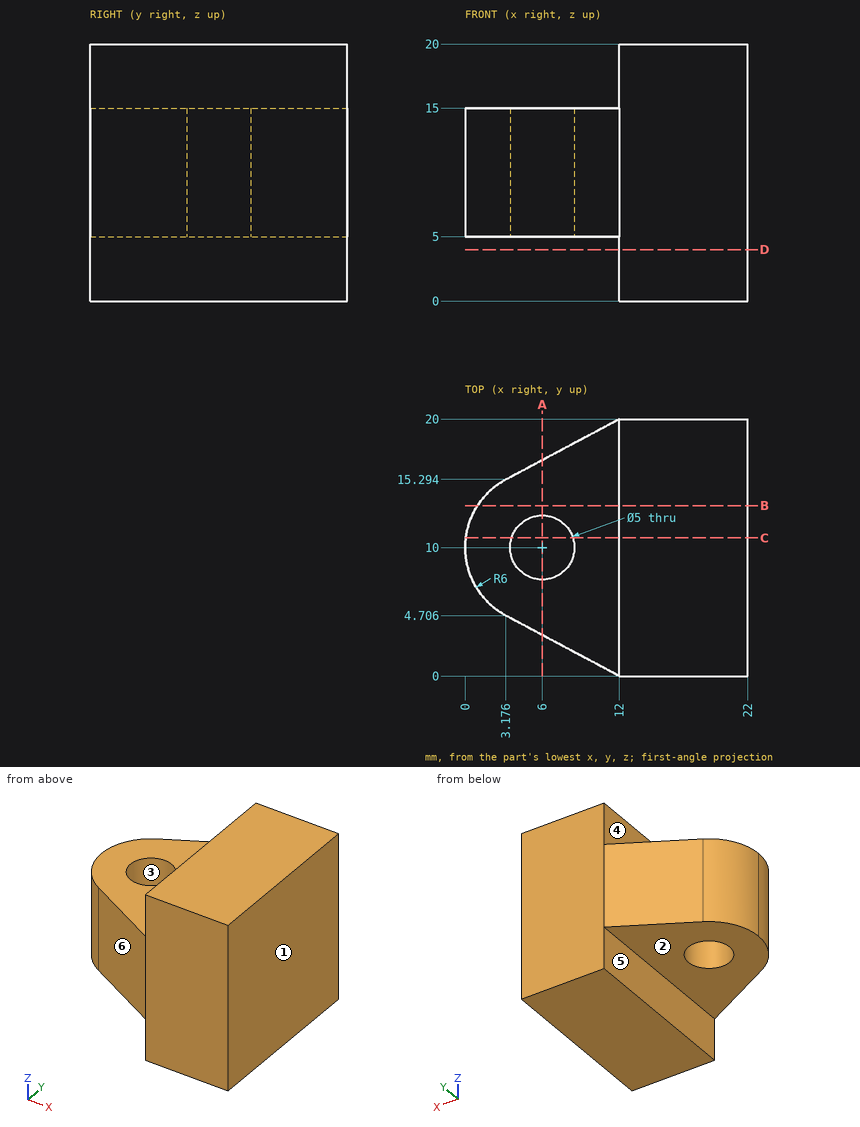
Design review of the part shown in the three views and the two pictorial views. Dimensions are in mm from the part's minimum x, y and z. A direction names the side the tool comes from. Round coordinates to 2 decimals unless told otherwise and drop trailing zeros. Order: outer loops, then holes, each group sorted by start corner. A loop starts at its lowest first (then second) coordinate and runs counter-clockwise, first axis right, second up.
(1) Mouldability with a two-part tool opening along X and no side actions: class the marked faces 1, 2 and 3 as released by +X, released by -X, zero draft, split by the parting line, or undercut.
Working result:
face 1: released by +X
face 2: zero draft
face 3: undercut
(2) Take a section at A-A, the plane x = 6. State the section outline as (y, z) points.
Working result:
outline: (3.2, 5) - (7.5, 5) - (7.5, 15) - (3.2, 15) - close; (12.5, 5) - (16.8, 5) - (16.8, 15) - (12.5, 15) - close
(3) Wall thickness on L1, parallel to Z at x = 10.5, y = 14.5; L2, parallel to Y at x = 7, z = 5.25 (1 decimal); L3, parallel to Y at x = 6, z = 9.5: over which ranges is each line inside the solid? List them lowest first.
Working result:
L1: z = 5 to 15
L2: y = 2.7 to 7.7, 12.3 to 17.3
L3: y = 3.2 to 7.5, 12.5 to 16.8
(4) Take a section at B-B, the plane y = 13.25. State the section outline as (x, z) points.
Working result:
outline: (0.96, 5) - (12, 5) - (12, 0) - (22, 0) - (22, 20) - (12, 20) - (12, 15) - (0.96, 15) - close
(5) Tool access review of the marked faces 4, 5 and 6: name each direction out of +Z, -Z, +X, -X, +Y, -Y from which nothing blocks a thin tool from reaching the whole face with its end or side.
Working result:
face 4: +Z, -X, +Y, -Y
face 5: -Z, -X, +Y, -Y
face 6: +Z, -Z, -X, -Y
(6) For P1, Ø6, axis at x = 8, y = 11, coming from the -Z side; P2, Ø6, axis at x = 3.5, y = 11, coming from the +Z side; P3, Ø5.5, axis at y = 6, z = 16.5, coming from the -X side (1 decimal), all flat-tipped, find the tip position at first contact; note any pin that passes through.
Working result:
P1: stops at z = 5
P2: stops at z = 15
P3: stops at x = 0.2
(7) Take a section at D-D, the plane z = 4. State the section outline as (x, y) points.
Working result:
outline: (12, 0) - (22, 0) - (22, 20) - (12, 20) - close
(8) Take a section at C-C, the plane y = 10.75. State the section outline as (x, z) points (1 decimal), plus the area to 3 significant figures.
Working result:
outline: (0, 5) - (3.6, 5) - (3.6, 15) - (0, 15) - close; (8.4, 5) - (12, 5) - (12, 0) - (22, 0) - (22, 20) - (12, 20) - (12, 15) - (8.4, 15) - close
area: 272 mm2
